Input: dimensioned drawing with shaded views. Units: mm. Origin: part minimum x, y, z. A direction names the side the tool comes from. Give positions to 0.01 mm unless a question says otherwise; leave off trailing zeros. Write each loop counter-clockwise with the first axis right and the second up, starting at its lowest first coordinate (ties: lowest second). Pieces come first, ordered by that corner, then holes. Notation, with made-up numbers: M -10,-8 L 40,-8 A14 ccw 40,1 Z; hole C -31.75,67 d2. An arc over 180 degrees is marked long. Use CSV: the item, a comma, the result in double quotes. Start each with the question number.
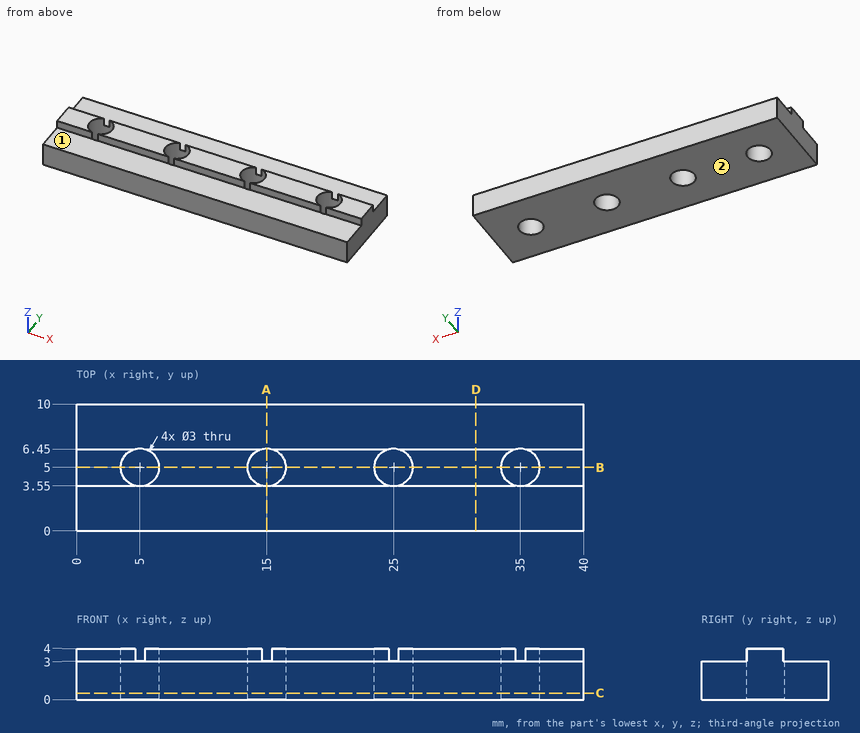
Q1. Section A-A, the plane x = 15. Return the cut outline in (y, z).
Q2. First-contact query: pin 1 Ø2.5 at (x, y) = (5, 5) entering from -Z; pin 2 Ø0.8 at (x, z) = (29, 3.5) entering from +Y; pin 3 Ø0.8 at (x, z) = (38, 3.5) entering from -Y; pin 4 Ø3 at (x, y) = (7, 2) entering from +Z. Flat tips, straight axial feed; report the tip coordinate or a pass-through.
Q3. Set-up query: the marked faces 1 and 2. Return all of +Z, -Z, +X, -X, +Y, -Y with unobstructed straight access to the full face (end or side cutting, diameter ignored); none if empty.
Q4. Section D-D, the plane x = 31.5. Return the cut outline in (y, z), and give its area (3 significant figures).
Q5. Section C-C, the plane z = 0.5. Return the cut outline in (x, y).
Q6. Material intervals for L1, parallel to Y at x = 35, z = 2.9; L2, parallel to X at y = 5.5, z = 1; L3, parallel to X at y = 5.75, z = 3.5, sorted ascending. Write a range as [from, to].
Q7. Section B-B, the plane y = 5. Return the cut outline in (x, z).
Check result:
1,outline,"M 0,0 L 3.5,0 L 3.5,3 L 0,3 Z; M 6.5,0 L 10,0 L 10,3 L 6.5,3 Z"
2,pin 1,"passes through"
2,pin 2,"stops at y = 6.45"
2,pin 3,"stops at y = 3.55"
2,pin 4,"stops at z = 3"
3,face 1,"+Z, +X, -X, -Y"
3,face 2,"-Z, +X, -X, +Y, -Y"
4,outline,"M 0,0 L 10,0 L 10,3 L 6.45,3 L 6.45,4 L 3.55,4 L 3.55,3 L 0,3 Z"
4,area,"32.9 mm²"
5,outline,"M 0,0 L 40,0 L 40,10 L 0,10 Z; hole C 5,5 d3; hole C 15,5 d3; hole C 25,5 d3; hole C 35,5 d3"
6,L1,"y = [0, 3.5], [6.5, 10]"
6,L2,"x = [0, 3.59], [6.41, 13.59], [16.41, 23.59], [26.41, 33.59], [36.41, 40]"
6,L3,"x = [0, 3.7], [6.3, 13.7], [16.3, 23.7], [26.3, 33.7], [36.3, 40]"
7,outline,"M 0,0 L 3.5,0 L 3.5,4 L 0,4 Z; M 6.5,0 L 13.5,0 L 13.5,4 L 6.5,4 Z; M 16.5,0 L 23.5,0 L 23.5,4 L 16.5,4 Z; M 26.5,0 L 33.5,0 L 33.5,4 L 26.5,4 Z; M 36.5,0 L 40,0 L 40,4 L 36.5,4 Z"
